Part print with two shaded views. Sizes in mm from the minimum x, y, z corner. Round coordinates to 2 decimals unless told otherwise and drop trailing zeros. Loops run counter-clockwise (first coordinate to the right, second up) from the corner with the lowest first, then second, coordinate; pieces in that order, holes last.
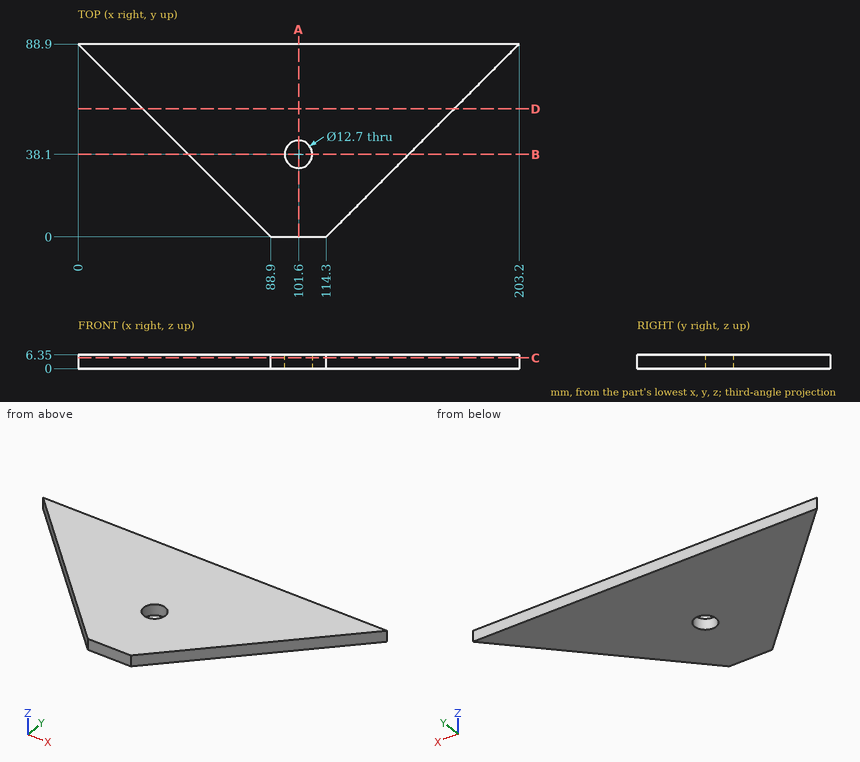
Item 1: Cut at A-A (x = 101.6). List the corners of the cut face in (y, z), plus the area to 3 significant figures.
Verdict:
outline: (0, 0) - (31.75, 0) - (31.75, 6.35) - (0, 6.35) - close; (44.45, 0) - (88.9, 0) - (88.9, 6.35) - (44.45, 6.35) - close
area: 484 mm2
Item 2: Flat gauge pins, fed straight in: P1, Ø3, axis at y = 58, z = 2.5, coming from the -X side; P2, Ø1, axis at x = 21, z = 4.5, coming from the -Y side; P3, Ø1, axis at y = 34, z = 5, coming from the -X side. Where does each tip first touch, or does it go through?
Verdict:
P1: stops at x = 29.4
P2: stops at y = 67.4
P3: stops at x = 54.4
Item 3: Cut at D-D (y = 59). List the corners of the cut face in (x, z).
Verdict:
outline: (29.9, 0) - (173.3, 0) - (173.3, 6.35) - (29.9, 6.35) - close
Item 4: Wall check: L1, parallel to Y at x = 101.6, z = 4.5; L2, parallel to Y at x = 98, z = 0.75; L3, parallel to X at y = 35, z = 6. Give the ranges that are in metal, low to high.
Verdict:
L1: y = 0 to 31.75, 44.45 to 88.9
L2: y = 0 to 32.87, 43.33 to 88.9
L3: x = 53.9 to 96.06, 107.14 to 149.3
Item 5: Cut at B-B (y = 38.1). List the corners of the cut face in (x, z), plus the area to 3 significant figures.
Verdict:
outline: (50.8, 0) - (95.25, 0) - (95.25, 6.35) - (50.8, 6.35) - close; (107.95, 0) - (152.4, 0) - (152.4, 6.35) - (107.95, 6.35) - close
area: 565 mm2
Item 6: Cut at C-C (z = 5). List the corners of the cut face in (x, y), plus the area to 3 significant figures.
Verdict:
outline: (0, 88.9) - (88.9, 0) - (114.3, 0) - (203.2, 88.9) - close; hole circle Ø12.7 at (101.6, 38.1)
area: 10,000 mm2
